Source: CAD feature listing. Evaluate the final solid. Frame: model axes, mm. Give positions to 0.01 mm unless a question says otherwise; leave off trailing zeros. Loops run counter-clockwise (first coordinate to the right, second up) from the corner with the lowest first, then second, coordinate; pieces in that order, holes last.
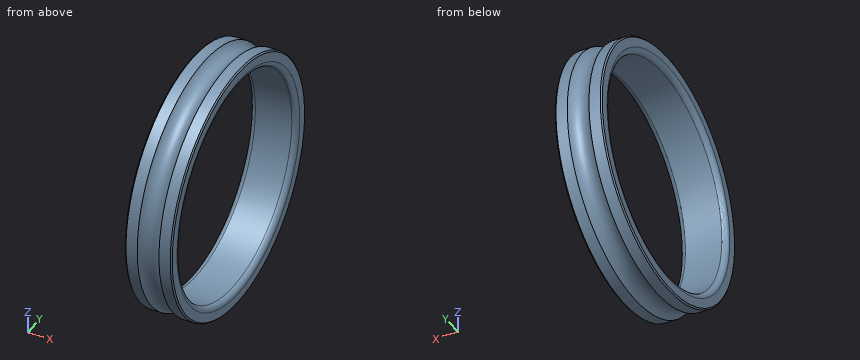
```python
from build123d import *

# Parameters (mm, degrees)
CHANFREIN2_SIZE = 0.5


with BuildPart() as part:
    # Esquisse1 → Base-Révolution (revolve)
    with BuildSketch(Plane.XY, mode=Mode.PRIVATE) as base_r_volution_sk:
        with BuildLine():
            Line((2, 42.5), (16, 42.5))
            ThreePointArc((16, 42.5), (17.414213562, 43.085786438), (18, 44.5))
            Line((18, 44.5), (18, 48.5))
            Line((18, 48.5), (13.175823272, 48.5))
            ThreePointArc((13.175823272, 48.5), (9, 46.25), (4.824176728, 48.5))
            Line((4.824176728, 48.5), (0, 48.5))
            Line((0, 48.5), (0, 44.5))
            ThreePointArc((0, 44.5), (0.585786438, 43.085786438), (2, 42.5))
        make_face()
    revolve(base_r_volution_sk.sketch.rotate(Axis((0, 0, 0), (1, 0, 0)), 90), axis=Axis((0, 0, 0), (1, 0, 0)))

    # Chanfrein2
    chanfrein2_edges = [part.edges().sort_by_distance(p)[0] for p in [
        (18, 0, -48.5),
        (0, 0, -48.5),
    ]]
    chamfer(chanfrein2_edges, length=CHANFREIN2_SIZE)


solid = part.part
```
(1) Section D-D, the plane x = 10.75. Return the cut outline in (y, z).
A:
outline: circle Ø93.13 at (0, 0); hole circle Ø85 at (0, 0)
(2) Section C-C, the plane x = 3.5. Return the cut outline in (y, z), then the cut area to 3 significant figures.
A:
outline: circle Ø97 at (0, 0); hole circle Ø85 at (0, 0)
area: 1,720 mm2
(3) Ray query, line 1 along Y through (x, z) = (8.25, -14.5); line 2 along Z through (x, y) = (14.25, -4.5); line 3 along Y through (x, z) = (9.5, 0). Return the intervals inside material, ascending.
A:
line 1: y = -43.98 to -39.95, 39.95 to 43.98
line 2: z = -48.29 to -42.26, 42.26 to 48.29
line 3: y = -46.28 to -42.5, 42.5 to 46.28
(4) First-contact query: pin 1 (12 mm diameter, centred on y = -36.5, z = -30, fed in from -X); pin 2 (10 mm diameter, centred on x = 9, z = 20.5, fed in from -Y); pin 3 (2 mm diameter, centred on x = 5.5, z = -35.5, fed in from +Y); pin 4 (3 mm diameter, centred on x = 6.5, y = -29, fed in from -Z). Flat tips, straight axial feed; report the tip coordinate or a pass-through.
A:
pin 1: stops at x = 0
pin 2: stops at y = -45.14
pin 3: stops at y = 33.82
pin 4: stops at z = -38.81
(5) Section A-A, the plane z = 0. Return the cut outline in (x, y).
A:
outline: (0, -48) - (0.5, -48.5) - (4.82, -48.5) arc R5 cw to (13.18, -48.5) - (17.5, -48.5) - (18, -48) - (18, -44.5) arc R2 ccw to (16, -42.5) - (2, -42.5) arc R2 ccw to (0, -44.5) - close; (0, 44.5) arc R2 ccw to (2, 42.5) - (16, 42.5) arc R2 ccw to (18, 44.5) - (18, 48) - (17.5, 48.5) - (13.18, 48.5) arc R5 cw to (4.82, 48.5) - (0.5, 48.5) - (0, 48) - close
